Verification items for the finished model (mm, model axes). Face numbers are marked on the shaded views. Coordinates: 2 decimals unless noted, no trailing zeros. Write each loop counter-clockwise with the first axis right and the second up, starting at its lowest first coordinate (ties: lowest second). Pieces come first, ordered by that corner, then holes. Notation, with made-up numbers: (81.5, 14) -> (117.5, 14) arc R9 ccw to (117.5, 20) -> close; hole circle Ø1 at (19, 53). An arc over 180 degrees is marked (long way). Answer in a Markdown table with one row per item.
```python
from build123d import *

# Parameters (mm, degrees)
F0_R     = 37
F1_DEPTH = 2.5
F2_R     = 37
F2_R_2   = 35
F3_DEPTH = 175


with BuildPart() as f1:
    # F0 (on Top) → F1 (new body)
    with BuildSketch(Plane.XY):
        Circle(F0_R)
        with BuildLine():
            Line((32.982701, -3.842347), (27.482701, -3.842347))
            ThreePointArc((27.482701, -3.842347), (-0.110238, -27.749781), (-27.512361, -3.623876))
            Line((-27.512361, -3.623876), (-32.939691, -3.623876))
            Line((-32.939691, -3.623876), (-32.939691, 3.876124))
            Line((-32.939691, 3.876124), (-27.477958, 3.876124))
            ThreePointArc((-27.477958, 3.876124), (0.110256, 27.749781), (27.507891, 3.657653))
            Line((27.507891, 3.657653), (32.982701, 3.657653))
            Line((32.982701, 3.657653), (32.982701, -3.842347))
        make_face(mode=Mode.SUBTRACT)
    extrude(amount=F1_DEPTH)

    # F2 (on face) → F3 (join)
    with BuildSketch(Plane.XY.offset(2.5)):
        Circle(F2_R)
        Circle(F2_R_2, mode=Mode.SUBTRACT)
    extrude(amount=F3_DEPTH)


solid = f1.part
```
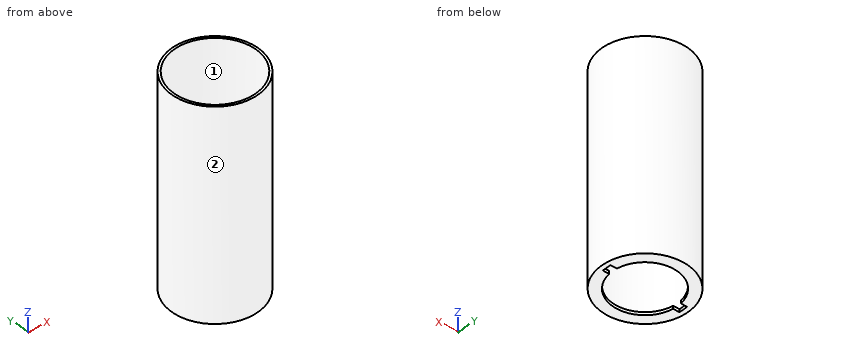
1. Section check C-C, the plane z = 94.5. Record the boundary of the cut face in (x, y), plus the area to 3 significant figures.
Geometry says:
| item | result |
|---|---|
| outline | circle Ø74 at (0, 0); hole circle Ø70 at (0, 0) |
| area | 452 mm^2 |
2. Section check A-A, the plane y = 0. Record the boundary of the cut face in (x, z).
Geometry says:
| item | result |
|---|---|
| outline | (-37, 0) -> (-32.94, 0) -> (-32.94, 2.5) -> (-35, 2.5) -> (-35, 177.5) -> (-37, 177.5) -> close; (32.98, 0) -> (37, 0) -> (37, 177.5) -> (35, 177.5) -> (35, 2.5) -> (32.98, 2.5) -> close |
3. Section check B-B, the plane x = 0. Record the boundary of the cut face in (y, z), plus the area to 3 significant figures.
Geometry says:
| item | result |
|---|---|
| outline | (-37, 0) -> (-27.75, 0) -> (-27.75, 2.5) -> (-35, 2.5) -> (-35, 177.5) -> (-37, 177.5) -> close; (27.75, 0) -> (37, 0) -> (37, 177.5) -> (35, 177.5) -> (35, 2.5) -> (27.75, 2.5) -> close |
| area | 746 mm^2 |
4. Mould release check, pull along X, two halves, no side actions. Record for the marked faces 1 and 2: released by +X, released by -X, zero draft, split by the parting line, or undercut.
Geometry says:
| item | result |
|---|---|
| face 1 | undercut |
| face 2 | split by the parting line |
5. Depth check by flat-ended pin: P1, Ø0.8, axis at x = 29.5, z = 1, coming from the -Y side; P2, Ø5, axis at x = -11, z = 110.5, coming from the -Y side; P3, Ø4, axis at y = 14, z = 33, coming from the +X side. Enter the tip coordinate at first touch or a pass-through.
Geometry says:
| item | result |
|---|---|
| P1 | y = -22.85 |
| P2 | y = -36.01 |
| P3 | x = 35 |
6. Thickness scan on line 1 (Y direction, x = 0, z = 57); line 2 (Y direction, x = -7.5, z = 42); line 3 (X direction, y = -22, z = 158). Record the ranges inside material, lowest first. Write a range as from..to.
Geometry says:
| item | result |
|---|---|
| line 1 | -37..-35, 35..37 |
| line 2 | -36.23..-34.19, 34.19..36.23 |
| line 3 | -29.75..-27.22, 27.22..29.75 |
